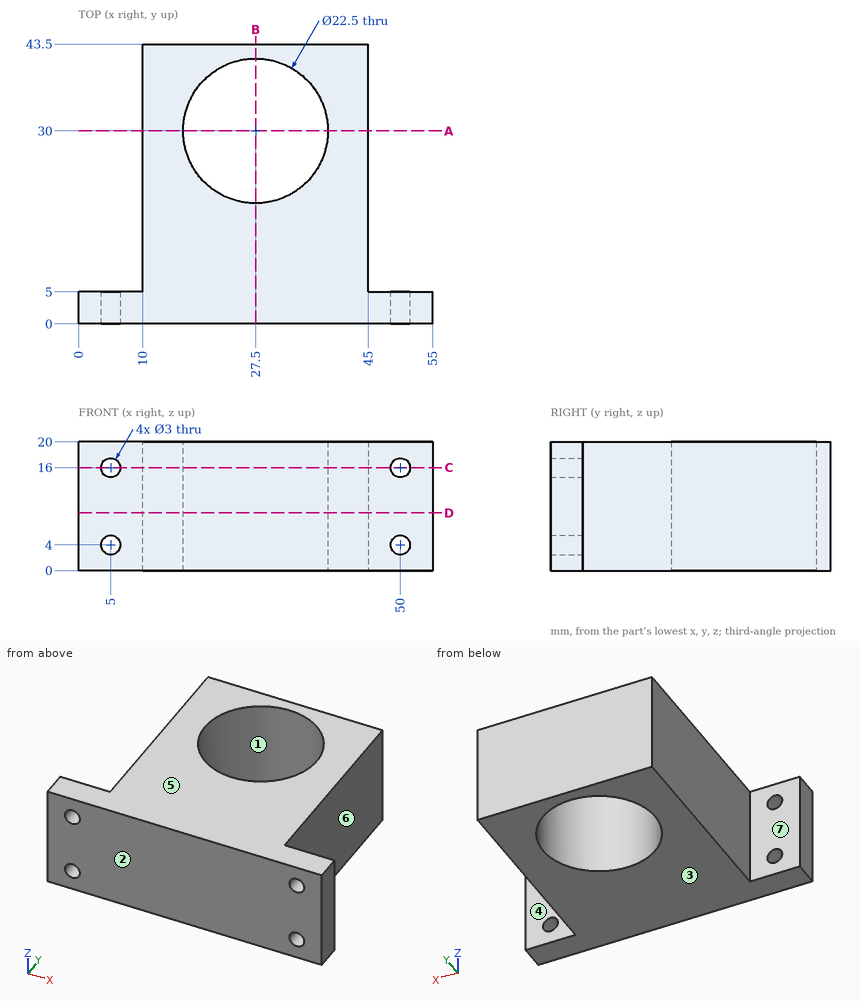
Could you check a few things on this drawing? It's one solid part, dimensions in mm from its lowest x, y, z. A direction names the side the tool comes from. Give positions to 0.01 mm unless a question says otherwise; leave off trailing zeros. Write each loop counter-clockwise with the first axis right and the second up, starting at its lowest first coordinate (ties: lowest second). Pieces come first, ordered by that corner, then holes. Notation, with made-up numbers: M 11,76.25 L 51,76.25 A12 ccw 51,86.25 Z; hole C 76,63 d10. An arc over 180 degrees is marked long. Put each result on its own line as item: value. Start each with the question number.
Item 1: I need wall thicknesses on L1, parallel to Z at x = 50, y = 3.05; L2, parallel to X at y = 3.05, z = 4; L3, parallel to Y at x = 27, z = 9. Which ranges of each line are inside material? Lowest first, please. Write a range as from..to.
Item 2: If we section it at D-D, the plane z = 9: Write out the boundary of the cut face in (x, y).
Item 3: If we section it at B-B, the plane x = 27.5: Write out the boundary of the cut face in (y, z), then the cut area to 3 significant figures.
Item 4: Thinking about a two-plate mould opening in Y: for the marked faces 1, 2, 3 and 4, which applies, +Y half, -Y half, draft (parallel to the pull), parting line (faces both ways), or undercut?
Item 5: Will these pins go through, and if not, where does the flat tip stop? pin 1 (3 mm diameter, centred on x = 3.5, z = 6, fed in from +Y); pin 2 (1 mm diameter, centred on y = 18.5, z = 14, fed in from +X); pin 3 (8 mm diameter, centred on y = 13, z = 15, fed in from -X).
Item 6: If we section it at A-A, the plane y = 30: Write out the boundary of the cut face in (x, z).
Item 7: If we section it at C-C, the plane z = 16: Write out the boundary of the cut face in (x, y), then the cut area to 3 significant figures.
Item 8: On a 3-axis mill with a long thin cutter (end or side, diameter ignored), from which of +Z, -Z, +X, -X, +Y, -Y can I reach the whole of each face in a straight line? I mean the marked faces 5, 6 and 7. Say none if no direction works.
Values:
1. L1: 0..2.5, 5.5..14.5, 17.5..20
1. L2: 0..3.5, 6.5..48.5, 51.5..55
1. L3: 0..18.76, 41.24..43.5
2. outline: M 0,0 L 55,0 L 55,5 L 45,5 L 45,43.5 L 10,43.5 L 10,5 L 0,5 Z; hole C 27.5,30 d22.5
3. outline: M 0,0 L 18.75,0 L 18.75,20 L 0,20 Z; M 41.25,0 L 43.5,0 L 43.5,20 L 41.25,20 Z
3. area: 420 mm²
4. face 1: undercut
4. face 2: -Y half
4. face 3: draft
4. face 4: +Y half
5. pin 1: y = 5
5. pin 2: x = 45
5. pin 3: x = 10
6. outline: M 10,0 L 16.25,0 L 16.25,20 L 10,20 Z; M 38.75,0 L 45,0 L 45,20 L 38.75,20 Z
7. outline: M 0,0 L 3.5,0 L 3.5,5 L 0,5 Z; M 6.5,0 L 48.5,0 L 48.5,5 L 45,5 L 45,43.5 L 10,43.5 L 10,5 L 6.5,5 Z; M 51.5,0 L 55,0 L 55,5 L 51.5,5 Z; hole C 27.5,30 d22.5
7. area: 1,190 mm²
8. face 5: +Z, +X, -X, +Y, -Y
8. face 6: +Z, -Z, +X, +Y
8. face 7: +Z, -Z, -X, +Y
